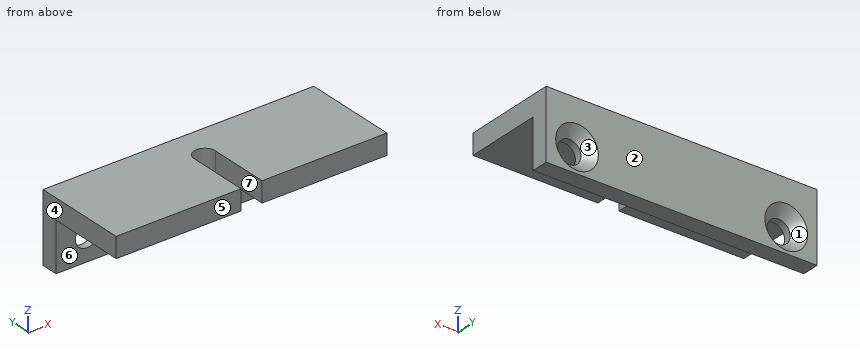
```python
from build123d import *

# Parameters (mm, degrees)
SKETCH1_W                                      = 40
SKETCH1_H                                      = 7.2
BOSS_EXTRUDE1_DEPTH                            = 2.5
CSK_FOR_M3_FLAT_HEAD_MACHINE_SCREW1_AT_2_COUNT = 2
CSK_FOR_M3_FLAT_HEAD_MACHINE_SCREW1_AT_2_PITCH = 30.9
SKETCH4_W                                      = 40
SKETCH4_H                                      = 3
BOSS_EXTRUDE2_DEPTH                            = 14
CUT_EXTRUDE1_DEPTH                             = 43.851954448


with BuildPart() as part:
    # Sketch1 → Boss-Extrude1 (new body)
    with BuildSketch(Plane(origin=(0, 0, 0), x_dir=(1, 0, 0), z_dir=(0, 1, 0))):
        with Locations((20, 3.6)):
            Rectangle(SKETCH1_W, SKETCH1_H)
    extrude(amount=BOSS_EXTRUDE1_DEPTH)

    # Sketch3 → CSK for M3 Flat Head Machine Screw1 (revolve, cut)
    with BuildSketch(Plane(origin=(35.45, 2.5, -3.6), x_dir=(0, 0, 1), z_dir=(1, 0, 0))):
        Polygon((0, 0), (0, 2.5), (1.7, 2.5), (1.7, 1.45), (3.15, 0), align=None)
    csk_for_m3_flat_head_machine_screw1 = revolve(axis=Axis((35.45, 8.85, -3.6), (0, -1, 0)), mode=Mode.SUBTRACT)

    # CSK for M3 Flat Head Machine Screw1 at 2: CSK for M3 Flat Head Machine Screw1 ×2
    with Locations(*[(-i * CSK_FOR_M3_FLAT_HEAD_MACHINE_SCREW1_AT_2_PITCH, 0, 0) for i in range(1, CSK_FOR_M3_FLAT_HEAD_MACHINE_SCREW1_AT_2_COUNT)]):
        add(csk_for_m3_flat_head_machine_screw1, mode=Mode.SUBTRACT)

    # Sketch4 → Boss-Extrude2 (add)
    with BuildSketch(Plane(origin=(0, 2.5, 0), x_dir=(1, 0, 0), z_dir=(0, 1, 0))):
        with Locations((20, -1.5)):
            Rectangle(SKETCH4_W, SKETCH4_H)
    extrude(amount=-BOSS_EXTRUDE2_DEPTH)

    # Sketch5 → Cut-Extrude1 (cut, through all)
    with BuildSketch(Plane.XY.offset(3)):
        with BuildLine():
            Line((18.45, -2.55), (18.45, -11.5))
            Line((18.45, -11.5), (21.55, -11.5))
            Line((21.55, -11.5), (21.55, -2.55))
            ThreePointArc((21.55, -2.55), (20, -1), (18.45, -2.55))
        make_face()
        with BuildLine():
            Line((21.55, -11.5), (18.45, -11.5))
            ThreePointArc((18.45, -11.5), (20, -13.05), (21.55, -11.5))
        make_face()
    extrude(amount=-CUT_EXTRUDE1_DEPTH, mode=Mode.SUBTRACT)


solid = part.part
```
Source: CAD feature listing. Evaluate the final solid. Frame: model axes, mm. Face numbers are marked on the shaded views. A direction names the side the tool comes from. Coordinates: 2 decimals unless noted, no trailing zeros. Order: outer loops, then holes, each group sorted by start corner. A loop starts at its lowest first (then second) coordinate and runs counter-clockwise, first axis right, second up. Notation, with made-up numbers: (43.25, -6) - (99.25, -6) arc R28 ccw to (99.25, 22) - close; hole circle Ø6 at (59.25, -27.75). An arc over 180 degrees is marked (long way). One line per item, written item: value.
1) Contact query for flat-ended pins moving along their axis: pin 1 (2.5 mm diameter, centred on x = 35.45, z = -3.6, fed in from -Y); pin 2 (1.5 mm diameter, centred on y = -6, z = 2, fed in from -X); pin 3 (1 mm diameter, centred on x = 27, y = -2.5, fed in from -Z); pin 4 (5.5 mm diameter, centred on x = 4.55, z = -3.6, fed in from -Y). Output: stop coordinate, or through.
Computed values:
pin 1: passes through
pin 2: stops at x = 0
pin 3: stops at z = 0
pin 4: stops at y = 0
2) Cut plane A-A on x = 35.45. Output: boundary loops of the cut face in (y, z), plus the area to 3 significant figures.
Computed values:
outline: (-11.5, 0) - (0, 0) - (0, -1.9) - (1.05, -1.9) - (2.5, -0.45) - (2.5, 3) - (-11.5, 3) - close; (0, -7.2) - (2.5, -7.2) - (2.5, -6.75) - (1.05, -5.3) - (0, -5.3) - close
area: 49.4 mm^2
3) Cut plane C-C on z = 0.75. Output: boundary loops of the cut face in (x, y), plus the area to 3 significant figures.
Computed values:
outline: (0, -11.5) - (18.45, -11.5) - (18.45, -2.55) arc R1.55 cw to (21.55, -2.55) - (21.55, -11.5) - (40, -11.5) - (40, 2.5) - (0, 2.5) - close
area: 528 mm^2
4) Ray query, line 1 (X direction, y = 0.4, z = -3.6); line 2 (Z direction, x = 35.45, y = 0.85); line 3 (X direction, y = -7.75, z = 0.5). Return the intervals inside material, ascending. Write a range as [from, to].
Computed values:
line 1: x = [0, 2.85], [6.25, 33.75], [37.15, 40]
line 2: z = [-7.2, -5.3], [-1.9, 3]
line 3: x = [0, 18.45], [21.55, 40]
5) Cut plane B-B on y = -5.5. Output: boundary loops of the cut face in (x, z), plus the area to 3 significant figures.
Computed values:
outline: (0, 0) - (18.45, 0) - (18.45, 3) - (0, 3) - close; (21.55, 0) - (40, 0) - (40, 3) - (21.55, 3) - close
area: 111 mm^2
6) Mould query, pull axis X, two halves, no side actions, for the marked faces 1, 2, 3 and 4. Classes: released by +X, released by -X, zero draft, split by the parting line, or undercut.
Computed values:
face 1: undercut
face 2: zero draft
face 3: undercut
face 4: released by -X
7) Cut plane D-D on y = 1.5. Output: boundary loops of the cut face in (x, z), plus the area to 3 significant figures.
Computed values:
outline: (0, -7.2) - (40, -7.2) - (40, 3) - (0, 3) - close; hole circle Ø4.3 at (4.55, -3.6); hole circle Ø4.3 at (35.45, -3.6)
area: 379 mm^2
8) Reachability of the marked faces 5, 6 and 7 from +Z, -Z, +X, -X, +Y, -Y: full face, straight path, thin tool, end or side. Return the list, or none.
Computed values:
face 5: +Z, -Z, +X, -X, -Y
face 6: -Z, +X, -X, -Y
face 7: +Z, -Z, -Y
